from build123d import *

# Parameters (mm, degrees)
SKETCH1_W           = 100
SKETCH1_H           = 100
SKETCH1_R           = 4
SKETCH1_R_2         = 15
BOSS_EXTRUDE1_DEPTH = 5
SKETCH2_R           = 2.5
CUT_EXTRUDE1_DEPTH  = 10


with BuildPart() as part:
    # Sketch1 → Boss-Extrude1 (new body)
    with BuildSketch(Plane.XY):
        with Locations((50, 50)):
            Rectangle(SKETCH1_W, SKETCH1_H)
        with Locations((15, 85)):
            Circle(SKETCH1_R, mode=Mode.SUBTRACT)
        with Locations((85, 85)):
            Circle(SKETCH1_R, mode=Mode.SUBTRACT)
        with Locations((85, 15)):
            Circle(SKETCH1_R, mode=Mode.SUBTRACT)
        with Locations((15, 15)):
            Circle(SKETCH1_R, mode=Mode.SUBTRACT)
        with Locations((50, 50)):
            Circle(SKETCH1_R_2, mode=Mode.SUBTRACT)
    extrude(amount=BOSS_EXTRUDE1_DEPTH)

    # Sketch2 → Cut-Extrude1 (cut)
    with BuildSketch(Plane.XY.offset(5)):
        with Locations((20, 72)):
            Circle(SKETCH2_R)
        with Locations((40, 72)):
            Circle(SKETCH2_R)
        with Locations((60, 72)):
            Circle(SKETCH2_R)
        with Locations((80, 72)):
            Circle(SKETCH2_R)
        with Locations((80, 28)):
            Circle(SKETCH2_R)
        with Locations((60, 28)):
            Circle(SKETCH2_R)
        with Locations((40, 28)):
            Circle(SKETCH2_R)
        with Locations((20, 28)):
            Circle(SKETCH2_R)
    extrude(amount=-CUT_EXTRUDE1_DEPTH, mode=Mode.SUBTRACT)


solid = part.part
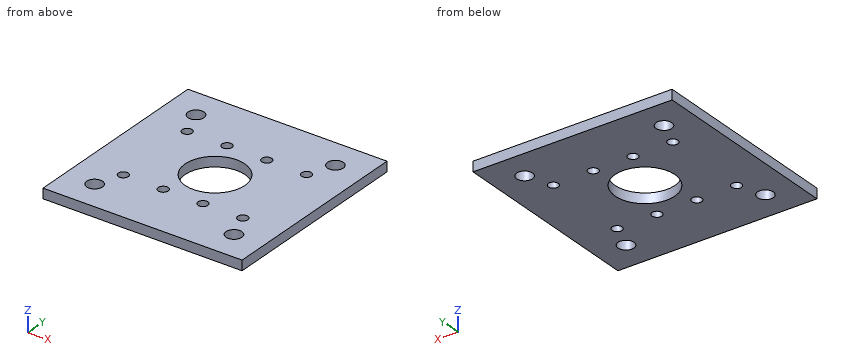
Work out the finished part from the listing and answer in its coordinate system (mm). Give positions to 0.01 mm unless a question says otherwise; leave off trailing zeros. Write each loop counter-clockwise with the first axis right and the second up, starting at its lowest first coordinate (ties: lowest second). Pieces come first, ordered by that corner, then holes.
Q1. Given pin 1 (9 mm diameter, centred on x = 15, y = 85, fed in from -Z), flat-ended and moving along its own axis, determine where the tip first touches the part or whether it passes through.
Answer:
pin 1: stops at z = 0
Q2. Straight lines are drawn through the part: L1, parallel to Y at x = 20, z = 3.9; L2, parallel to Y at x = 11.5, z = 4.45; L3, parallel to Y at x = 50, z = 2.1. For each, find the intervals that lie inside material, in ascending order.
Answer:
L1: y = 0 to 25.5, 30.5 to 69.5, 74.5 to 100
L2: y = 0 to 13.06, 16.94 to 83.06, 86.94 to 100
L3: y = 0 to 35, 65 to 100
Q3. The part is cut by section C-C on z = 0.8. State how many separate pieces and enclosed holes the cut face has, and give its area (4 significant figures).
Answer:
separate pieces: 1
enclosed holes: 13
area: 8,935 mm2
Q4. The part is cut by section D-D on x = 50. Give the vertices of the cut face in (y, z), and give its area (3 significant figures).
Answer:
outline: (0, 0) - (35, 0) - (35, 5) - (0, 5) - close; (65, 0) - (100, 0) - (100, 5) - (65, 5) - close
area: 350 mm2
Q5. The part is cut by section A-A on x = 85. Give the vertices of the cut face in (y, z), and give its area (3 significant figures).
Answer:
outline: (0, 0) - (11, 0) - (11, 5) - (0, 5) - close; (19, 0) - (81, 0) - (81, 5) - (19, 5) - close; (89, 0) - (100, 0) - (100, 5) - (89, 5) - close
area: 420 mm2
